Geometry check sheet. Reference: drawing and pictorial views, mm from the part's lowest x, y, z. Coordinates: 2 decimals unless noted, no trailing zeros. Write each loop counter-clockwise with the first axis right and the second up, starting at its lowest first coordinate (ties: lowest second). Pieces come first, ordered by that corner, then holes.
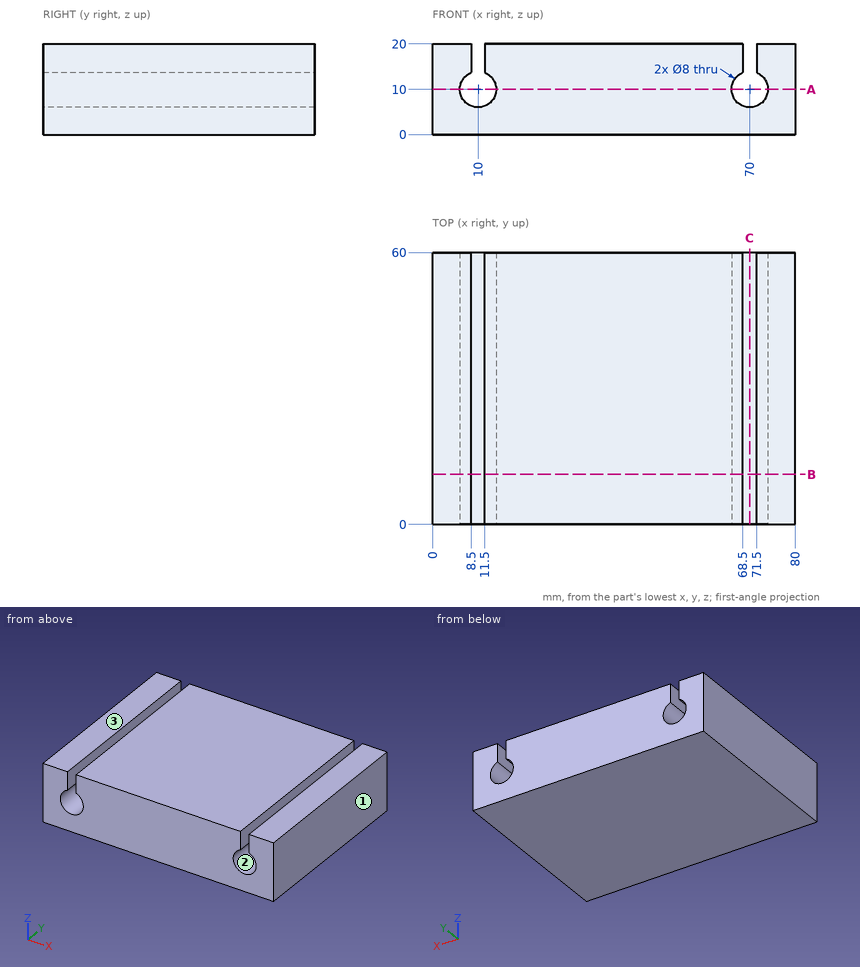
1. Draft check along X on the marked faces 1, 2 and 3. Enter one of: pulls with the +X half, pulls with the -X half, needs draft (parallel to the pull), parting line crosses it, or undercut.
2. Material ranges on L1, parallel to X at y = 54, z = 9.75; L2, parallel to X at y = 51, z = 14.75; L3, parallel to Z at x = 69, y = 13, recorded low to high.
3. Sectioned sample at C-C, the plane x = 70. Record the boundary of the cut face in (y, z).
4. Sectioned sample at B-B, the plane y = 11. Record the boundary of the cut face in (x, z).
5. Sectioned sample at A-A, the plane z = 10. Record the boundary of the cut face in (x, y), and give its area (3 significant figures).
Outcome:
1. face 1: pulls with the +X half
1. face 2: undercut
1. face 3: needs draft
2. L1: x = 0 to 6.01, 13.99 to 66.01, 73.99 to 80
2. L2: x = 0 to 8.5, 11.5 to 68.5, 71.5 to 80
2. L3: z = 0 to 6.13
3. outline: (0, 0) - (60, 0) - (60, 6) - (0, 6) - close
4. outline: (0, 0) - (80, 0) - (80, 20) - (71.5, 20) - (71.5, 13.71) arc R4 cw (long way) to (68.5, 13.71) - (68.5, 20) - (11.5, 20) - (11.5, 13.71) arc R4 cw (long way) to (8.5, 13.71) - (8.5, 20) - (0, 20) - close
5. outline: (0, 0) - (6, 0) - (6, 60) - (0, 60) - close; (14, 0) - (66, 0) - (66, 60) - (14, 60) - close; (74, 0) - (80, 0) - (80, 60) - (74, 60) - close
5. area: 3,840 mm2
